Verification items for the finished model (mm, model axes). Round coordinates to 2 decimals unless told otherwise and drop trailing zeros. Loops run counter-clockwise (first coordinate to the right, second up) from the corner with the lowest first, then second, coordinate; pieces in that order, holes last. Notation, with made-up numbers: (28, 7) -> (84, 7) arc R10 ccw to (84, 16) -> close; hole circle Ø9 at (-5, 32). An arc over 180 degrees is marked (long way). Use CSV: the item, a comma, the result in double quotes. Start each with the question number.
```python
from build123d import *

# Parameters (mm, degrees)
SKETCH_1_W      = 200
SKETCH_1_H      = 200
SKETCH_1_R      = 2
SKETCH_1_R_2    = 85
EXTRUDE_1_DEPTH = 4
FILLET_1_R      = 40
CHAMFER_1_SIZE  = 1


with BuildPart() as part:
    # Эскиз1 → Бобышка-Вытянуть1 (new body)
    with BuildSketch(Plane(origin=(0, 0, 0), x_dir=(1, 0, 0), z_dir=(0, 1, 0))):
        Rectangle(SKETCH_1_W, SKETCH_1_H)
        with Locations(Location((-85, 85, 0), (0, 0, 270))):
            Circle(SKETCH_1_R, mode=Mode.SUBTRACT)
        with Locations(Location((85, 85, 0), (0, 0, 270))):
            Circle(SKETCH_1_R, mode=Mode.SUBTRACT)
        with Locations(Location((85, -85, 0), (0, 0, 270))):
            Circle(SKETCH_1_R, mode=Mode.SUBTRACT)
        with Locations(Location((-85, -85, 0), (0, 0, 270))):
            Circle(SKETCH_1_R, mode=Mode.SUBTRACT)
        with Locations(Location((-90, 0, 0), (0, 0, 270))):
            Circle(SKETCH_1_R, mode=Mode.SUBTRACT)
        with Locations(Location((90, 0, 0), (0, 0, 90))):
            Circle(SKETCH_1_R, mode=Mode.SUBTRACT)
        with Locations(Location((75, 82, 0), (0, 0, 270))):
            Circle(SKETCH_1_R, mode=Mode.SUBTRACT)
        with Locations(Location((-75, 82, 0), (0, 0, 270))):
            Circle(SKETCH_1_R, mode=Mode.SUBTRACT)
        with Locations(Location((75, -82, 0), (0, 0, 270))):
            Circle(SKETCH_1_R, mode=Mode.SUBTRACT)
        with Locations(Location((-75, -82, 0), (0, 0, 270))):
            Circle(SKETCH_1_R, mode=Mode.SUBTRACT)
        with Locations(Location((82, -75, 0), (0, 0, 270))):
            Circle(SKETCH_1_R, mode=Mode.SUBTRACT)
        with Locations(Location((-82, -75, 0), (0, 0, 270))):
            Circle(SKETCH_1_R, mode=Mode.SUBTRACT)
        with Locations(Location((-82, 75, 0), (0, 0, 270))):
            Circle(SKETCH_1_R, mode=Mode.SUBTRACT)
        with Locations(Location((81.987312617, 75.001883036, 0), (0, 0, 270))):
            Circle(SKETCH_1_R, mode=Mode.SUBTRACT)
        with Locations(Location((0, 0, 0), (0, 0, 270))):
            Circle(SKETCH_1_R_2, mode=Mode.SUBTRACT)
    extrude(amount=EXTRUDE_1_DEPTH)

    # Скругление1
    fillet_1_edges = [part.edges().sort_by_distance(p)[0] for p in [
        (100, 2, 100),
        (-100, 2, 100),
        (-100, 2, -100),
        (100, 2, -100),
    ]]
    fillet(fillet_1_edges, radius=FILLET_1_R)

    # Фаска1
    chamfer_1_edges = [part.edges().sort_by_distance(p)[0] for p in [
        (-100, 0, 0),
        (-100, 4, 0),
        (100, 0, 0),
        (0, 0, 100),
        (0, 0, -100),
        (88.284271247, 0, 88.284271247),
        (88.284271247, 0, -88.284271247),
        (-88.284271247, 0, 88.284271247),
        (-88.284271247, 0, -88.284271247),
        (0, 4, -100),
        (100, 4, 0),
        (0, 4, 100),
        (88.284271247, 4, 88.284271247),
        (88.284271247, 4, -88.284271247),
        (-88.284271247, 4, 88.284271247),
        (-88.284271247, 4, -88.284271247),
    ]]
    chamfer(chamfer_1_edges, length=CHAMFER_1_SIZE)


solid = part.part
```
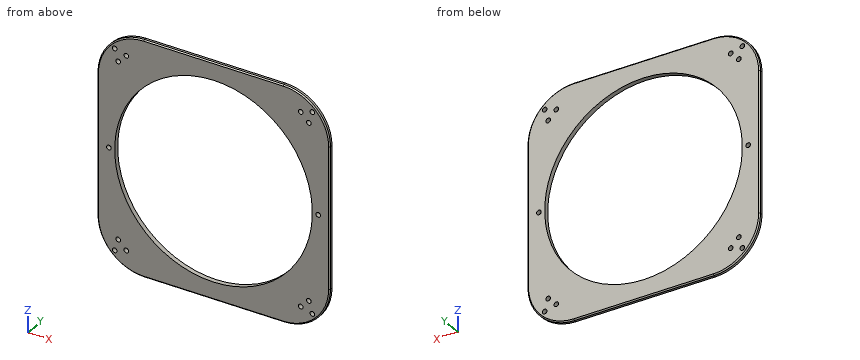
Q1. Thickness scan on L1, parallel to X at y = 2.55, z = 75; L2, parallel to X at y = 0.8, z = -91; L3, parallel to X at y = 3.1, z = 23. Record the ranges inside material, lowest first. Write a range as from..to.
Q2. Cross-section at B-B (z = 29). Record the boundary of the cut face in (x, y).
Q3. Cross-section at A-A (x = 0). Record the boundary of the cut face in (y, z), and give its area (3 significant figures).
Q4. Cross-section at C-C (y = 2.1). State how many separate pieces and enclosed holes the cut face has, and give its area (3 significant figures).
Q5. Depth check by flat-ended pin: pin 1 Ø2.5 at (x, z) = (-82, -75) entering from +Y; pin 2 Ø4.5 at (x, z) = (-85, -85) entering from +Y. Enter the tip coordinate at first touch or a pass-through.
Answer list:
1,L1,"x = -97.08..-84, -80..-40, 40..80, 84..97.08"
1,L2,"x = -84.96..84.96"
1,L3,"x = -99.9..-81.83, 81.83..99.9"
2,outline,"(-100, 1) -> (-99, 0) -> (-79.9, 0) -> (-79.9, 4) -> (-99, 4) -> (-100, 3) -> close; (79.9, 0) -> (99, 0) -> (100, 1) -> (100, 3) -> (99, 4) -> (79.9, 4) -> close"
3,outline,"(0, -99) -> (1, -100) -> (3, -100) -> (4, -99) -> (4, -85) -> (0, -85) -> close; (0, 85) -> (4, 85) -> (4, 99) -> (3, 100) -> (1, 100) -> (0, 99) -> close"
3,area,"118 mm2"
4,separate pieces,"1"
4,enclosed holes,"15"
4,area,"15,800 mm2"
5,pin 1,"passes through"
5,pin 2,"stops at y = 4"
